CAD build for the part. Positions are in the model's coordinates, mm. Round coordinates to 2 decimals unless told otherwise and drop trailing zeros. Order: outer loops, then holes, each group sorted by start corner. A loop starts at its lowest first (then second) coordinate and runs counter-clockwise, first axis right, second up. Notation, with made-up numbers: (50, 20.25) - (108, 20.25) arc R13 cw to (108, 31.25) - close; hole circle Ø6 at (63, 39.25). An arc over 180 degrees is marked (long way). Write item = value, one per line.
from build123d import *

# Parameters (mm, degrees)
BOSS_EXTRUDE1_DEPTH = 7.2
SKETCH2_W           = 89.9
SKETCH2_H           = 148
BOSS_EXTRUDE2_DEPTH = 23.4
SKETCH3_W           = 12.2
SKETCH3_H           = 53.8
SKETCH3_W_2         = 12.4
SKETCH3_H_2         = 34.48
CUT_EXTRUDE1_DEPTH  = 9.9
SKETCH4_W           = 89.9
SKETCH4_H           = 3.586904051
SKETCH4_W_2         = 90
SKETCH4_H_2         = 2.297698364
CUT_EXTRUDE2_DEPTH  = 9.9
SKETCH5_W           = 18
SKETCH5_H           = 10
SKETCH5_W_2         = 13.128765808
SKETCH5_W_3         = 13.081709299
BOSS_EXTRUDE3_DEPTH = 13


with BuildPart() as part:
    # Sketch1 → Boss-Extrude1 (new body)
    with BuildSketch(Plane(origin=(0, 0, 0), x_dir=(1, 0, 0), z_dir=(0, 1, 0))):
        with BuildLine():
            Line((43, -85), (-43, -85))
            ThreePointArc((-43, -85), (-44.414213562, -84.414213562), (-45, -83))
            Line((-45, -83), (-45, 83))
            ThreePointArc((-45, 83), (-44.414213562, 84.414213562), (-43, 85))
            Line((-43, 85), (43, 85))
            ThreePointArc((43, 85), (44.414213562, 84.414213562), (45, 83))
            Line((45, 83), (45, -83))
            ThreePointArc((45, -83), (44.414213562, -84.414213562), (43, -85))
        make_face()
    extrude(amount=BOSS_EXTRUDE1_DEPTH)

    # Sketch2 → Boss-Extrude2 (add)
    with BuildSketch(Plane(origin=(0, 7.2, 0), x_dir=(1, 0, 0), z_dir=(0, 1, 0))):
        with Locations((0, 0.976122618)):
            Rectangle(SKETCH2_W, SKETCH2_H)
    extrude(amount=BOSS_EXTRUDE2_DEPTH)

    # Sketch3 → Cut-Extrude1 (cut)
    with BuildSketch(Plane(origin=(0, 30.6, 0), x_dir=(1, 0, 0), z_dir=(0, 1, 0))):
        with Locations((-38.85, -2.560293939)):
            Rectangle(SKETCH3_W, SKETCH3_H)
        with Locations((38.75, -6.331083764)):
            Rectangle(SKETCH3_W_2, SKETCH3_H_2)
    extrude(amount=-CUT_EXTRUDE1_DEPTH, mode=Mode.SUBTRACT)

    # Sketch4 → Cut-Extrude2 (cut)
    with BuildSketch(Plane(origin=(0, 30.6, 0), x_dir=(1, 0, 0), z_dir=(0, 1, 0))):
        with Locations((0, 67.894969538)):
            Rectangle(SKETCH4_W, SKETCH4_H)
        with Locations((0, 11.148849182)):
            Rectangle(SKETCH4_W_2, SKETCH4_H_2)
        with Locations((0, 16.148849182)):
            Rectangle(SKETCH4_W_2, SKETCH4_H_2)
        with Locations((0, 21.148849182)):
            Rectangle(SKETCH4_W_2, SKETCH4_H_2)
        with Locations((0, 26.148849182)):
            Rectangle(SKETCH4_W_2, SKETCH4_H_2)
        with Locations((0, 31.148849182)):
            Rectangle(SKETCH4_W_2, SKETCH4_H_2)
        with Locations((0, 36.148849182)):
            Rectangle(SKETCH4_W_2, SKETCH4_H_2)
        with Locations((0, 41.148849182)):
            Rectangle(SKETCH4_W_2, SKETCH4_H_2)
        with Locations((0, -41.148849182)):
            Rectangle(SKETCH4_W_2, SKETCH4_H_2)
        with Locations((0, -36.148849182)):
            Rectangle(SKETCH4_W_2, SKETCH4_H_2)
        with Locations((0, -31.148849182)):
            Rectangle(SKETCH4_W_2, SKETCH4_H_2)
        with Locations((0, -26.148849182)):
            Rectangle(SKETCH4_W_2, SKETCH4_H_2)
        with Locations((0, -21.148849182)):
            Rectangle(SKETCH4_W_2, SKETCH4_H_2)
        with Locations((0, -16.148849182)):
            Rectangle(SKETCH4_W_2, SKETCH4_H_2)
        with Locations((0, -11.148849182)):
            Rectangle(SKETCH4_W_2, SKETCH4_H_2)
        with Locations((0, -67.894969538)):
            Rectangle(SKETCH4_W, SKETCH4_H)
    extrude(amount=-CUT_EXTRUDE2_DEPTH, mode=Mode.SUBTRACT)

    # Sketch5 → Boss-Extrude3 (add)
    with BuildSketch(Plane(origin=(0, 7.2, 0), x_dir=(1, 0, 0), z_dir=(0, 1, 0))):
        with Locations((-35.870753406, -80.05)):
            Rectangle(SKETCH5_W, SKETCH5_H)
        with Locations((-16.922452044, -80.05)):
            Rectangle(SKETCH5_W, SKETCH5_H)
        with Locations((2.025849319, -80.05)):
            Rectangle(SKETCH5_W, SKETCH5_H)
        with Locations((18.149473412, -80.05)):
            Rectangle(SKETCH5_W_2, SKETCH5_H)
        with Locations((31.866445574, -80.05)):
            Rectangle(SKETCH5_W_3, SKETCH5_H)
        with Locations((31.866445574, 80.05)):
            Rectangle(SKETCH5_W_3, SKETCH5_H)
        with Locations((18.149473412, 80.05)):
            Rectangle(SKETCH5_W_2, SKETCH5_H)
        with Locations((2.025849319, 80.05)):
            Rectangle(SKETCH5_W, SKETCH5_H)
        with Locations((-16.922452044, 80.05)):
            Rectangle(SKETCH5_W, SKETCH5_H)
        with Locations((-35.870753406, 80.05)):
            Rectangle(SKETCH5_W, SKETCH5_H)
    extrude(amount=BOSS_EXTRUDE3_DEPTH)


solid = part.part
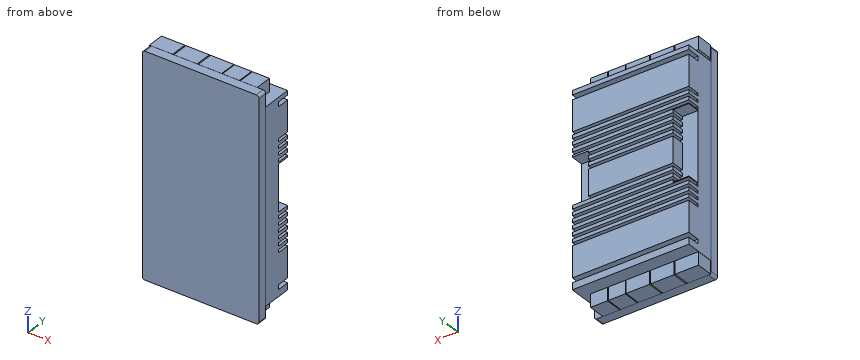
(1) Drop flat-ended pins along their axis: pin 1 (8 mm diameter, centred on y = 16, z = 82, fed in from +X); pin 2 (8 mm diameter, centred on x = -29.5, y = 24.5, fed in from +Z); pin 3 (4 mm diameter, centred on y = 21.5, z = 35, fed in from -X). Give the stop position or say it passes through.
Solved:
pin_1 = 38.41
pin_2 = 73.02
pin_3 = -44.95
(2) Band-saw the part on B-B on y = 23.5. Count the separate pieces of the cut face and the enclosed holes in it, plus the area to 3 significant figures.
Solved:
separate_pieces = 17
enclosed_holes = 0
area = 8,980 mm²
(3) Band-saw the part on A-A on z = 68. List the corners of the cut face in (x, y).
Solved:
outline = (-45, 0) - (45, 0) - (45, 7.2) - (44.95, 7.2) - (44.95, 20.7) - (-44.95, 20.7) - (-44.95, 7.2) - (-45, 7.2) - close
(4) Probe line 1 along X through (y, z) = (14.5, -10); line 2 along X through (y, z) = (21.5, -4); line 3 along Y through (x, z) = (-41, 11). List the from-to ranges inside material, lowest first.
Solved:
line_1 = -44.95 to 44.95
line_2 = -32.75 to 32.55
line_3 = 0 to 20.7
